Source: three-view drawing plus pictorial views. Frame: mm from the lowest corner of the part. Coordinates: 2 decimals unless noted, no trailing zeros. Loops run counter-clockwise (first coordinate to the right, second up) from the corner with the lowest first, then second, coordinate; pieces in that order, holes last. Notation, with made-up numbers: (49.25, -11) - (64.25, -11) arc R16 cw to (64.25, 20) - close; hole circle Ø6 at (81, 67). An arc over 180 degrees is marked (long way). Return JSON: item names as keys, results as strings.
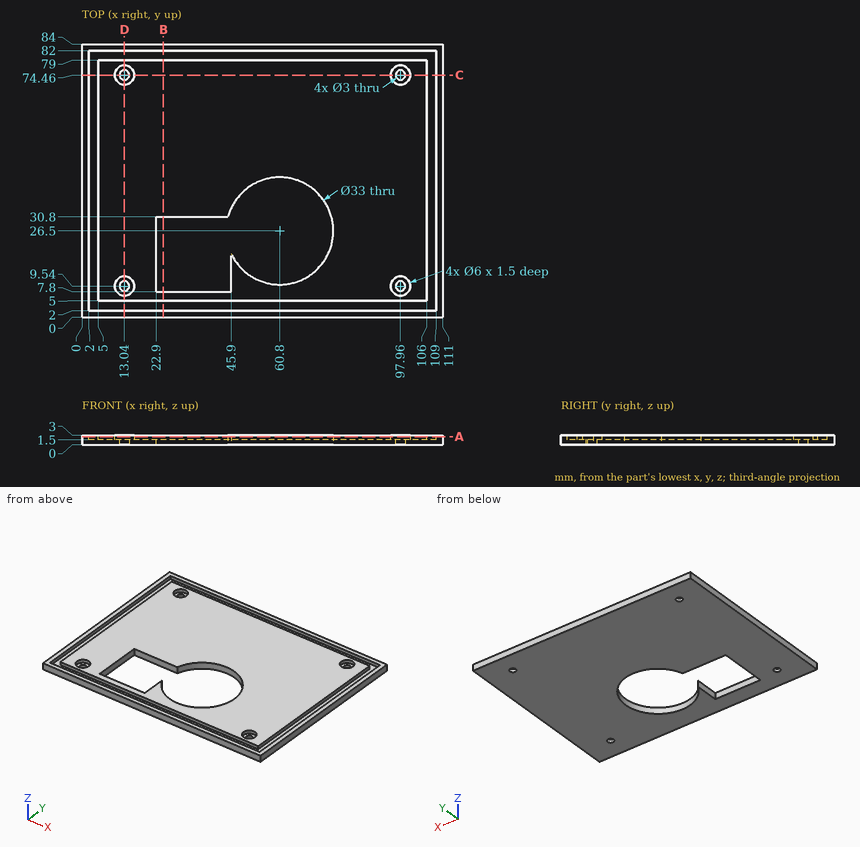
Item 1: Ray query, probe 1 along Y at (x, z) = (13.04, 2); probe 2 along X at (y, z) = (9.54, 2.55); probe 3 along X at (y, z) = (52, 2.6). Return the intervals inside material, ascending. Write a range as from..to.
Worked out:
{"probe 1": "0..2, 5..6.54, 12.54..71.46, 77.46..79, 82..84", "probe 2": "0..2, 5..10.04, 16.04..22.9, 45.9..94.96, 100.96..106, 109..111", "probe 3": "0..2, 5..106, 109..111"}
Item 2: Section query B-B, the plane x = 25. Return loops of the section in (y, z), and give its area (3 significant figures).
Worked out:
{"outline": "(0, 0) - (7.8, 0) - (7.8, 3) - (5, 3) - (5, 1.5) - (2, 1.5) - (2, 3) - (0, 3) - close; (30.8, 0) - (84, 0) - (84, 3) - (82, 3) - (82, 1.5) - (79, 1.5) - (79, 3) - (30.8, 3) - close", "area": "174 mm^2"}
Item 3: Section query A-A, the plane z = 2.5. Return loops of the section in (x, y), and give its area (3 significant figures).
Worked out:
{"outline": "(0, 0) - (111, 0) - (111, 84) - (0, 84) - close; (5, 5) - (106, 5) - (106, 79) - (5, 79) - close; hole (2, 2) - (109, 2) - (109, 82) - (2, 82) - close; hole circle Ø6 at (13.04, 9.54); hole circle Ø6 at (13.04, 74.46); hole (22.9, 7.8) - (45.9, 7.8) - (45.9, 19.41) arc R16.5 ccw (long way) to (44.87, 30.8) - (22.9, 30.8) - close; hole circle Ø6 at (97.96, 9.54); hole circle Ø6 at (97.96, 74.46)", "area": "6,750 mm^2"}
Item 4: Section query C-C, the plane y = 74.46. Return loops of the section in (x, z), and give its area (3 significant figures).
Worked out:
{"outline": "(0, 0) - (11.54, 0) - (11.54, 1.5) - (10.04, 1.5) - (10.04, 3) - (5, 3) - (5, 1.5) - (2, 1.5) - (2, 3) - (0, 3) - close; (14.54, 0) - (96.46, 0) - (96.46, 1.5) - (94.96, 1.5) - (94.96, 3) - (16.04, 3) - (16.04, 1.5) - (14.54, 1.5) - close; (99.46, 0) - (111, 0) - (111, 3) - (109, 3) - (109, 1.5) - (106, 1.5) - (106, 3) - (100.96, 3) - (100.96, 1.5) - (99.46, 1.5) - close", "area": "297 mm^2"}
Item 5: Section query D-D, the plane x = 13.04. Return loops of the section in (y, z).
Worked out:
{"outline": "(0, 0) - (8.04, 0) - (8.04, 1.5) - (6.54, 1.5) - (6.54, 3) - (5, 3) - (5, 1.5) - (2, 1.5) - (2, 3) - (0, 3) - close; (11.04, 0) - (72.96, 0) - (72.96, 1.5) - (71.46, 1.5) - (71.46, 3) - (12.54, 3) - (12.54, 1.5) - (11.04, 1.5) - close; (75.96, 0) - (84, 0) - (84, 3) - (82, 3) - (82, 1.5) - (79, 1.5) - (79, 3) - (77.46, 3) - (77.46, 1.5) - (75.96, 1.5) - close"}
Item 6: First-contact query: pin 1 Ø3.5 at (x, y) = (13.04, 74.46) entering from +Z; pin 2 Ø8 at (x, y) = (34.5, 23.5) entering from -Z. Flat tips, straight axial feed; report the tip coordinate or a pass-through.
Worked out:
{"pin 1": "z = 1.5", "pin 2": "through"}
